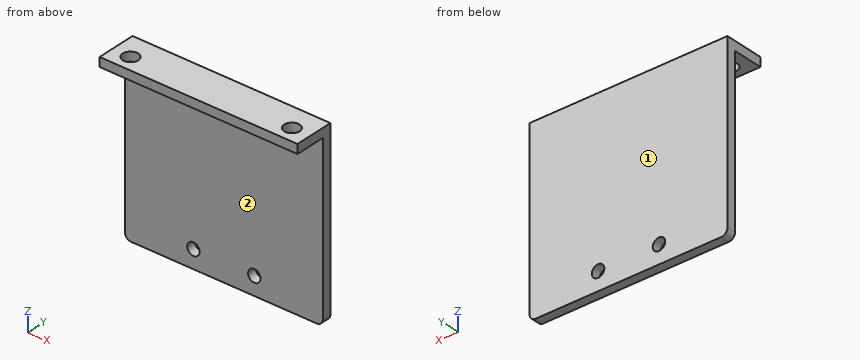
```python
from build123d import *

# Parameters (mm, degrees)
F0_W     = 65
F0_H     = 59
F1_DEPTH = 3
F2_W     = 65
F2_H     = 3
F3_DEPTH = 10
F4_R     = 2.55
F5_DEPTH = 25
F6_R     = 2.05
F7_DEPTH = 25
F8_R     = 2


with BuildPart() as f1:
    # F0 (on Front) → F1 (new body)
    with BuildSketch(Plane.XZ):
        with Locations((32.5, -29.5)):
            Rectangle(F0_W, F0_H)
    extrude(amount=F1_DEPTH)

    # F2 (on face) → F3 (join)
    with BuildSketch(Plane.XZ.offset(3)):
        with Locations((32.5, -1.5)):
            Rectangle(F2_W, F2_H)
    extrude(amount=F3_DEPTH)

    # F4 (on face) → F5 (cut)
    with BuildSketch(Plane.XY):
        with Locations((59.0165, -8)):
            Circle(F4_R)
        with Locations((5.9835, -8)):
            Circle(F4_R)
    extrude(amount=-F5_DEPTH, mode=Mode.SUBTRACT)

    # F6 (on face) → F7 (cut)
    with BuildSketch(Plane(origin=(0, 0, 0), x_dir=(-1, 0, 0), z_dir=(0, 1, 0))):
        with Locations((-42.5, -53)):
            Circle(F6_R)
        with Locations((-22.5, -53)):
            Circle(F6_R)
    extrude(amount=-F7_DEPTH, mode=Mode.SUBTRACT)

    # F8
    f8_edges = [f1.edges().sort_by_distance(p)[0] for p in [
        (65, -1.5, -59),
        (0, -1.5, -59),
    ]]
    fillet(f8_edges, radius=F8_R)


solid = f1.part
```
For this review, take the finished solid that the model builds, in its own axes (mm). Face numbers are marked on the shaded views. A direction names the side the tool comes from. Give positions to 0.01 mm unless a question says otherwise; leave off trailing zeros. Write each loop counter-clockwise with the first axis right and the second up, starting at its lowest first coordinate (ties: lowest second). Pieces come first, ordered by that corner, then holes.
Item 1: Take a section at D-D (x = 38.5). Give the boundary of the cut face in (y, z).
Item 2: Machinability: for the marked faces 1 and 2, which of the approach directions +Z, -Z, +X, -X, +Y, -Y give a long, thin tool a straight path to every point of the face, cutting with its end or side? Answer none if there is none.
Item 3: Take a section at C-C (y = -8). Give the boundary of the cut face in (x, z), and give its area (3 significant figures).
Item 4: Take a section at B-B (z = -53). Give the boundary of the cut face in (x, y).
Item 5: Take a section at A-A (x = 22.5). Give the boundary of the cut face in (y, z), and give its area (3 significant figures).
Item 6: Insertion check: P1, Ø5.5, axis at x = 22.5, z = -53, coming from the -Y side; P2, Ø4, axis at x = 36, y = -11.5, coming from the -Z side. Each pin has a flat end and moves straight along its axis. Give the tip position at first contact, or say it passes through.
Item 7: Wall thickness on probe 1 along Y at (x, z) = (10, -10): over which ranges is the line inside the solid? List them lowest first.
Established:
1. outline: (-13, -3) - (-3, -3) - (-3, -59) - (0, -59) - (0, 0) - (-13, 0) - close
2. face 1: +Z, -Z, +X, -X, +Y
2. face 2: -Z, +X, -X, -Y
3. outline: (0, -3) - (3.43, -3) - (3.43, 0) - (0, 0) - close; (8.53, -3) - (56.47, -3) - (56.47, 0) - (8.53, 0) - close; (61.57, -3) - (65, -3) - (65, 0) - (61.57, 0) - close
3. area: 164 mm2
4. outline: (0, -3) - (20.45, -3) - (20.45, 0) - (0, 0) - close; (24.55, -3) - (40.45, -3) - (40.45, 0) - (24.55, 0) - close; (44.55, -3) - (65, -3) - (65, 0) - (44.55, 0) - close
5. outline: (-13, -3) - (-3, -3) - (-3, -50.95) - (0, -50.95) - (0, 0) - (-13, 0) - close; (-3, -59) - (0, -59) - (0, -55.05) - (-3, -55.05) - close
5. area: 195 mm2
6. P1: stops at y = -3
6. P2: stops at z = -3
7. probe 1: y = -3 to 0
